Here's the drawing with two shaded views (mm, measured from the low corner). I have some questions. Give positions to 0.01 mm unless a question says otherwise; leave off trailing zeros. Loops run counter-clockwise (first coordinate to the right, second up) from the corner with the lowest first, then second, coordinate; pieces in that order, holes last. Notation, with made-up numbers: M -34,40 L -9,40 A7 cw -9,47 Z; hole C -37,-38.75 d9. An arc over 180 degrees is marked long. Answer in a Markdown table with one row per item. Add a question column.
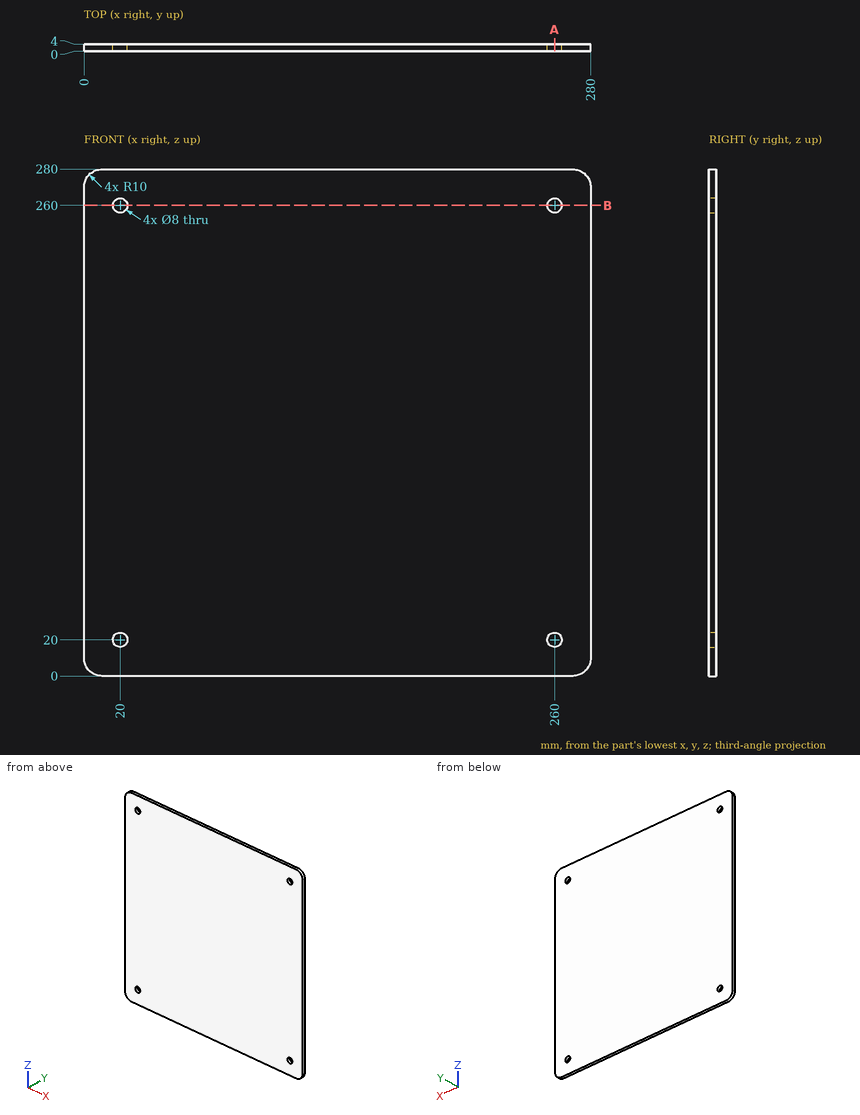
Item 1: For P1, Ø7, axis at x = 20, z = 20, coming from the +Y side, with a flat end and sliding along its axis, tell me the tip position at first contact or that it passes through.
Item 2: Suppose I cut it at A-A (x = 260). List the corners of the cut face in (y, z) for me.
Item 3: I need wall thicknesses on L1, parallel to Z at x = 260, y = 3; L2, parallel to X at y = 1.25, z = 259. Which ranges of each line are inside material? Lowest first, please.
Item 4: Suppose I cut it at B-B (z = 260). List the corners of the cut face in (x, y) for me, then the cut area to 3 significant figures.
Values found:
| question | item | result |
|---|---|---|
| 1 | P1 | through |
| 2 | outline | M 0,0 L 4,0 L 4,16 L 0,16 Z; M 0,24 L 4,24 L 4,256 L 0,256 Z; M 0,264 L 4,264 L 4,280 L 0,280 Z |
| 3 | L1 | 0 to 16, 24 to 256, 264 to 280 |
| 3 | L2 | 0 to 16.13, 23.87 to 256.13, 263.87 to 280 |
| 4 | outline | M 0,0 L 16,0 L 16,4 L 0,4 Z; M 24,0 L 256,0 L 256,4 L 24,4 Z; M 264,0 L 280,0 L 280,4 L 264,4 Z |
| 4 | area | 1,060 mm² |
